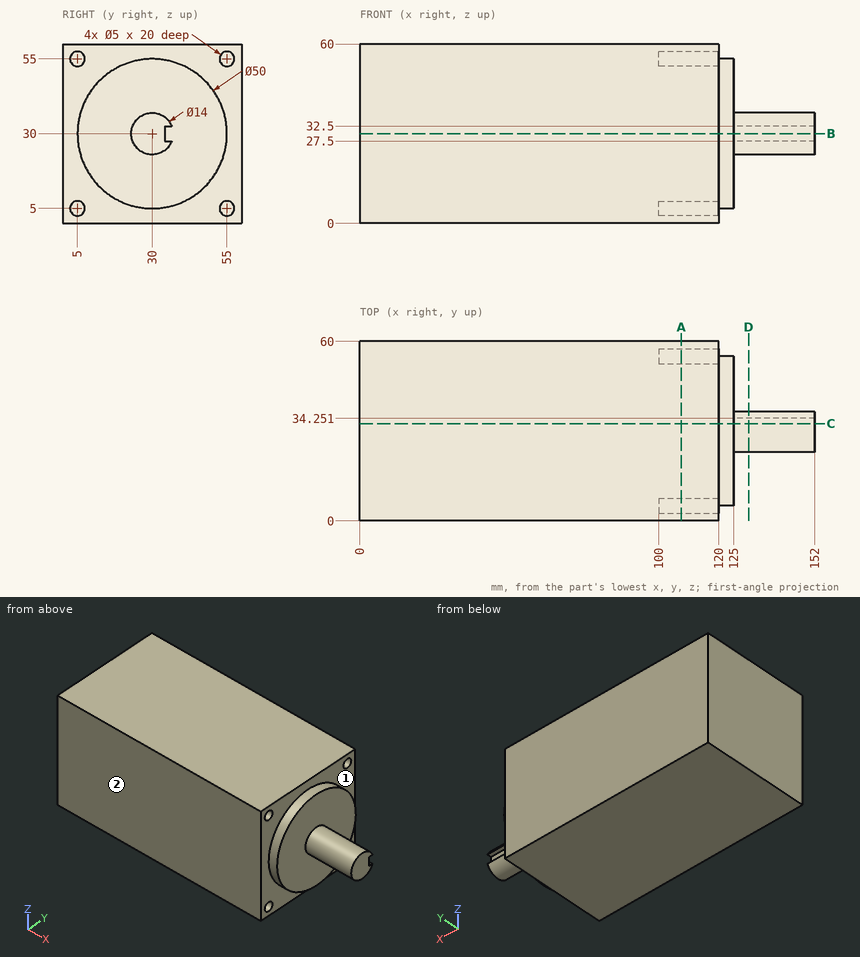
The drawing under review shows one solid part. Ordinate dimensions are in mm from its lowest x, y, z. A direction names the side the tool comes from. Coordinates: 2 decimals unless noted, no trailing zeros. Order: outer loops, then holes, each group sorted by start corner. A loop starts at its lowest first (then second) coordinate and runs counter-clockwise, first axis right, second up. Notation, with made-up numbers: (87.25, 16) -> (125.25, 16) arc R31 ccw to (125.25, 45) -> close; hole circle Ø3 at (-30, 23.5). An arc over 180 degrees is marked (long way). Answer in a Markdown table with one row per item. Add a question column.
Item 1: We need section C-C on y = 32.5. Write out the cut boundary in (x, z) (1 decimal).
Item 2: We need section A-A on x = 107.5. Write out the cut boundary in (y, z), plus the area to 3 significant figures.
Item 3: We need section D-D on x = 130. Write out the cut boundary in (y, z), plus the area to 3 significant figures.
Item 4: Machinability: for the marked faces 1 and 2, which of the approach directions +Z, -Z, +X, -X, +Y, -Y give a long, thin tool a straight path to every point of the face, cutting with its end or side? Answer none if there is none.
Item 5: To check wall thickness, follow probe 1 along Y at (x, z) = (110.5, 55); probe 2 along X at (y, z) = (23.5, 26.5); probe 3 along X at (y, z) = (5, 33). State the ranges of each line that lie inside material, in increasing order.
Item 6: We need section B-B on z = 30. Write out the cut boundary in (x, y), plus the area to 3 significant figures.
Item 7: Clearance check with flat-ended pins moving along their axes: pin 1 (4 mm diameter, centred on y = 5.5, z = 6, fed in from +X); pin 2 (1.8 mm diameter, centred on x = 132, y = 35.5, fed in from +Z); pin 3 (2.5 mm diameter, centred on y = 54.5, z = 54.5, fed in from +X). State where each tip first meets the part, or that it passes through.
Final values:
| question | item | result |
|---|---|---|
| 1 | outline | (0, 0) -> (120, 0) -> (120, 5.1) -> (125, 5.1) -> (125, 23.5) -> (152, 23.5) -> (152, 36.5) -> (125, 36.5) -> (125, 54.9) -> (120, 54.9) -> (120, 60) -> (0, 60) -> close |
| 2 | outline | (0, 0) -> (60, 0) -> (60, 60) -> (0, 60) -> close; hole circle Ø5 at (5, 5); hole circle Ø5 at (5, 55); hole circle Ø5 at (55, 5); hole circle Ø5 at (55, 55) |
| 2 | area | 3,520 mm2 |
| 3 | outline | (34.25, 27.5) -> (34.25, 32.5) -> (36.54, 32.5) arc R7 ccw (long way) to (36.54, 27.5) -> close |
| 3 | area | 141 mm2 |
| 4 | face 1 | +X |
| 4 | face 2 | +Z, -Z, +X, -X, -Y |
| 5 | probe 1 | y = 0 to 2.5, 7.5 to 52.5, 57.5 to 60 |
| 5 | probe 2 | x = 0 to 125 |
| 5 | probe 3 | x = 0 to 120 |
| 6 | outline | (0, 0) -> (120, 0) -> (120, 5) -> (125, 5) -> (125, 23) -> (152, 23) -> (152, 34.25) -> (125, 34.25) -> (125, 55) -> (120, 55) -> (120, 60) -> (0, 60) -> close |
| 6 | area | 7,750 mm2 |
| 7 | pin 1 | stops at x = 120 |
| 7 | pin 2 | stops at z = 35.28 |
| 7 | pin 3 | stops at x = 100 |
